Part print with two shaded views. Sizes in mm from the minimum x, y, z corner. Give positions to 0.01 mm unless a question says otherwise; leave off trailing zeros. Write each loop counter-clockwise with the first axis right and the second up, starting at its lowest first coordinate (ties: lowest second). Pieces come first, ordered by that corner, then holes. Notation, with made-up numbers: (23, 85) - (55, 85) arc R24 cw to (55, 104) - close; hole circle Ø10 at (17, 12). An arc over 180 degrees is marked (long way). Answer as a JSON object with one key per item and string values. Group by question number.
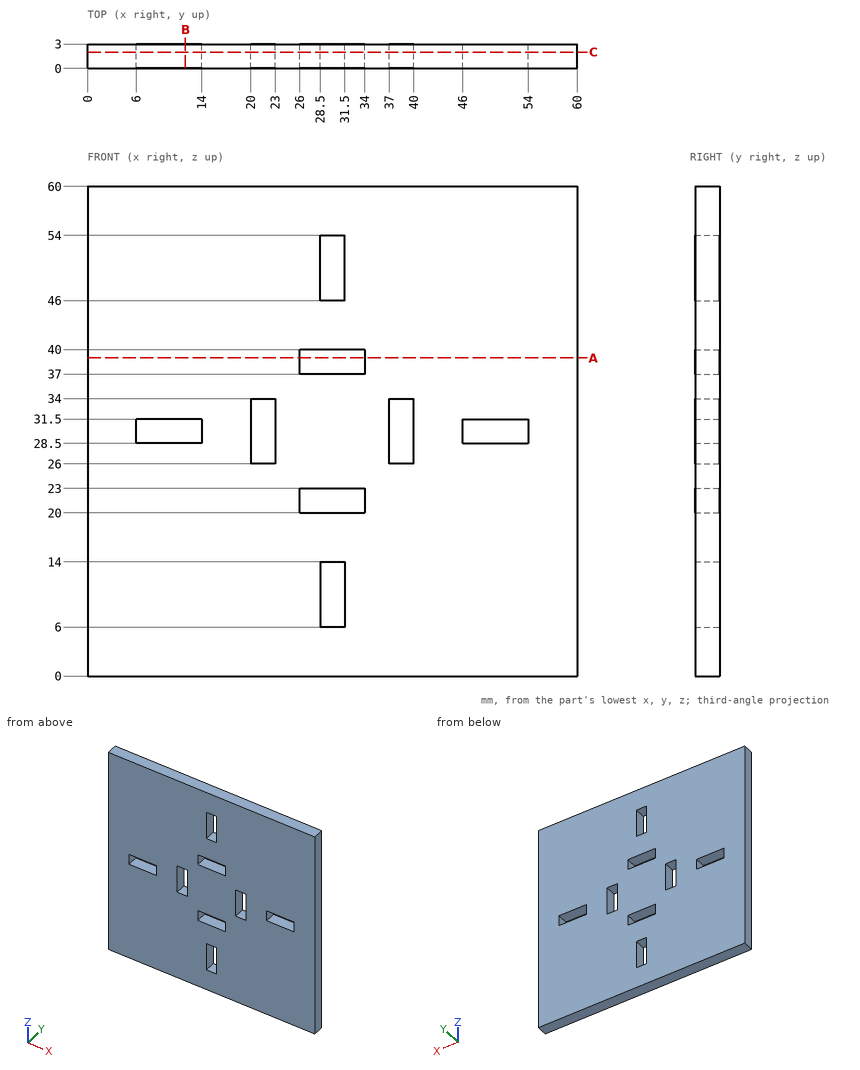
1) Drop a flat-ended pin along its axis: P1, Ø0.9, axis at y = 2, z = 30, coming from the -X side. Give the stop position or say it passes through.
2) Saw through at C-C (y = 2). State how many separate pieces and enclosed holes the cut face has, and give its area (3 significant figures).
3) Saw through at B-B (x = 12). List the corners of the cut face in (y, z).
4) Saw through at A-A (z = 39). List the corners of the cut face in (x, y).
5) Drill centre lines: line 1 along X through (y, z) = (2.55, 29); line 2 along Z through (x, y) = (33, 1.75). Where is each one in solid material? Low to high. Write a range as from..to.
Checks:
{
 "1": {"P1": "x = 0"},
 "2": {"separate pieces": "1", "enclosed holes": "8", "area": "3,410 mm2"},
 "3": {"outline": "(0, 0) - (3, 0) - (3, 28.5) - (0, 28.5) - close; (0, 31.5) - (3, 31.5) - (3, 60) - (0, 60) - close"},
 "4": {"outline": "(0, 0) - (26, 0) - (26, 3) - (0, 3) - close; (34, 0) - (60, 0) - (60, 3) - (34, 3) - close"},
 "5": {"line 1": "0..6, 14..20, 23..37, 40..46, 54..60", "line 2": "0..20, 23..37, 40..60"}
}
